The model under review builds one solid part; all positions refer to its coordinate system, in mm. Face numbers are marked on the shaded views. A direction names the side the tool comes from. Give positions to 0.01 mm unless a question says otherwise; leave off trailing zeros. Loops run counter-clockwise (first coordinate to the right, second up) from the corner with the lowest first, then second, coordinate; pieces in that order, holes last. Notation, with made-up numbers: M 31.5,81 L 77.5,81 A17 cw 77.5,97 Z; hole C -17,61 d4. An arc over 180 degrees is marked long. Write item = value, one per line. Start each with the question number.
1. For pin 1 (12 mm diameter, centred on x = -6.5, y = 6, fed in from -Z); pin 2 (8.5 mm diameter, centred on y = -1, z = -27, fed in from +X); pin 3 (1 mm diameter, centred on x = -2, y = 3, fed in from +Z); pin 4 (6 mm diameter, centred on y = -2, z = -7.5, fed in from +X), all flat-tipped, find the tip position at first contact; note any pin that passes through.
2. Draft analysis for pull direction Y (two halves, no side actions). For the marked faces 3, 4, 5 and 6, state which applies: pulls with the +Y half, pulls with the -Y half, needs draft (parallel to the pull), parting line crosses it, or undercut.
3. For the marked faces 1 and 2, list the 3-axis set-ups (+Z, -Z, +X, -X, +Y, -Y) from which the entire face can be reached by the end or side of a thin tool; tool diameter is ignored.
4. We need section D-D on z = -42. Give the boundary of the cut face in (x, y).
5. We need section B-B on y = 0. Count the separate pieces of the cut face and the enclosed holes in it, then the cut area to 3 significant figures.
6. Wall thickness on line 1 along X through (y, z) = (3, -35); line 2 along Z through (x, y) = (-5.25, 0); line 3 along Y through (x, z) = (8.75, -18): over which ranges is each line inside the solid? List them lowest first. Write a range as from..to.
7. We need section A-A on z = -17. Give the boundary of the cut face in (x, y).
from build123d import *

# Parameters (mm, degrees)
F0_R      = 13.15
F0_R_2    = 10.15
F1_DEPTH  = 20
F2_R      = 8
F3_DEPTH  = 22.5
F4_R      = 40.4098259217
F4_R_2    = 13.15
F5_DEPTH  = 50
F6_W      = 2
F6_H      = 35
F7_DEPTH  = 31.2572
F8_SIZE   = 1.5
F9_R      = 1.55
F10_DEPTH = 30.51178
F12_DEPTH = 1.5


with BuildPart() as f1:
    # F0 (on Top) → F1 (new body)
    with BuildSketch(Plane.XY):
        Circle(F0_R)
        Circle(F0_R_2, mode=Mode.SUBTRACT)
    extrude(amount=-F1_DEPTH)

    # F2 (on Front) → F3 (join, symmetric)
    with BuildSketch(Plane.XZ):
        with BuildLine():
            ThreePointArc((-11, -35), (0, -46), (11, -35))
            ThreePointArc((11, -35), (0, -24), (-11, -35))
        make_face()
        with Locations((0, -35)):
            Circle(F2_R, mode=Mode.SUBTRACT)
        with BuildLine():
            ThreePointArc((-11, -35), (0, -24), (11, -35))
            Line((11, -35), (11, -24.0798275918))
            ThreePointArc((11, -24.0798275918), (11.5703901789, -21.7739929718), (13.15, -20))
            Line((13.15, -20), (-13.15, -20))
            ThreePointArc((-13.15, -20), (-11.5703901789, -21.7739929718), (-11, -24.0798275918))
            Line((-11, -24.0798275918), (-11, -35))
        make_face()
    extrude(amount=F3_DEPTH, both=True)

    # F4 (on face) → F5 (cut)
    with BuildSketch(Plane.XY):
        Circle(F4_R)
        Circle(F4_R_2, mode=Mode.SUBTRACT)
    extrude(amount=-F5_DEPTH, mode=Mode.SUBTRACT)

    # F6 (on face) → F7 (cut)
    with BuildSketch(Plane.XY):
        Rectangle(F6_W, F6_H)
    extrude(amount=-F7_DEPTH, mode=Mode.SUBTRACT)

    # F8
    f8_edges = [f1.edges().sort_by_distance(p)[0] for p in [
        (-13.15, 0, 0),
        (9.64553, 8.937911, 0),
        (9.64553, -8.937911, 0),
    ]]
    chamfer(f8_edges, length=F8_SIZE)

    # F9 (on face) → F10 (cut, symmetric)
    with BuildSketch(Plane(origin=(-11, 0, 0), x_dir=(0, -1, 0), z_dir=(-1, 0, 0))):
        with Locations((0, -25)):
            Circle(F9_R)
        with Locations((0, -8)):
            Circle(F9_R)
    extrude(amount=F10_DEPTH, both=True, mode=Mode.SUBTRACT)

    # F11 (on face) → F12 (cut, symmetric)
    with BuildSketch(Plane.YZ.offset(11)):
        Polygon((1.5877132403, -22.25), (-1.5877132403, -22.25), (-3.1754264805, -25), (-1.5877132403, -27.75), (1.5877132403, -27.75), (3.1754264805, -25), align=None)
    extrude(amount=F12_DEPTH, both=True, mode=Mode.SUBTRACT)


solid = f1.part
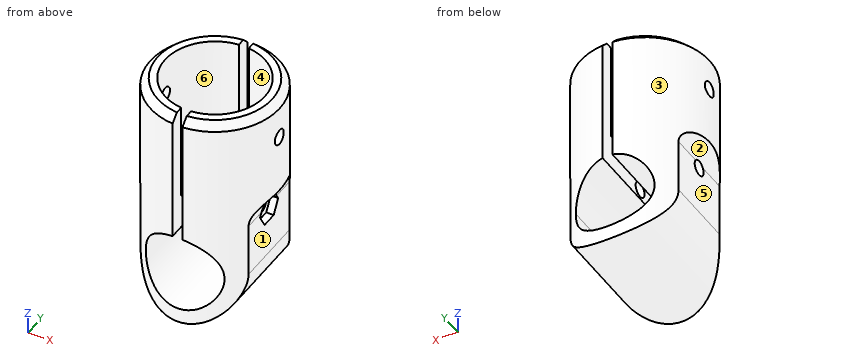
Final values:
q1.pin_1 = -45.99
q1.pin_2 = 11.15
q1.pin_3 = -20
q1.pin_4 = 13.15
q2.face_3 = parting line crosses it
q2.face_4 = undercut
q2.face_5 = needs draft
q2.face_6 = undercut
q3.face_1 = -Z, +X, +Y, -Y
q3.face_2 = -Z, -X, +Y, -Y
q4.outline = M -8.49,-10.05 A13.15 ccw -3.87,-12.57 L -3.87,12.57 A13.15 ccw -8.49,10.05 Z; M 3.87,-12.57 A13.15 ccw 8.49,-10.05 L 8.49,10.05 A13.15 ccw 3.87,12.57 Z
q5.separate_pieces = 5
q5.enclosed_holes = 0
q5.area = 344 mm²
q6.line_1 = -11..-8, 8..11
q6.line_2 = -44.67..-41.04, -28.96..-26.55, -23.45..-20
q6.line_3 = -9.82..-5.14, 5.14..9.82
q7.outline = M -1,-13.11 L -1,-10.1 A10.15 cw -1,10.1 L -1,13.11 A13.15 ccw Z; M 1,-13.11 A13.15 ccw 1,13.11 L 1,10.1 A10.15 cw 1,-10.1 Z
